```python
from build123d import *

# Parameters (mm, degrees)
EXTRUDE_1_DEPTH  = 11.2
SKETCH_3_W       = 40
SKETCH_3_H       = 20
EXTRUDE_2_DEPTH  = 5
EXTRUDE_3_DEPTH  = 10
EXTRUDE_4_DEPTH  = 5
SKETCH_7_W       = 98.8
SKETCH_7_H       = 34.24
EXTRUDE_5_DEPTH  = 9.8
SKETCH_8_W       = 80
SKETCH_8_H       = 34.24
EXTRUDE_6_DEPTH  = 5
SKETCH_9_W       = 35
SKETCH_9_H       = 30
EXTRUDE_7_DEPTH  = 5
EXTRUDE_8_DEPTH  = 40
FILLET_1_R       = 2
EXTRUDE_9_REACH  = 25.8
SKETCH_14_W      = 10
SKETCH_14_H      = 60
EXTRUDE_12_DEPTH = 167.8
EXTRUDE_13_DEPTH = 17.12
FILLET_3_R       = 2


with BuildPart() as part:
    # Sketch 1 → Extrude 1 (new body)
    with BuildSketch(Plane.XY):
        Polygon((0, 103.73), (5, 108.73), (95, 108.73), (100, 103.73), (100, 0), (0, 0), align=None)
    extrude(amount=EXTRUDE_1_DEPTH)



with BuildPart() as body_2:
    # Sketch 3 → Extrude 2 (new body)
    with BuildSketch(Plane.XY.offset(21.2)):
        with Locations((80, 86.29)):
            Rectangle(SKETCH_3_W, SKETCH_3_H)
    extrude(amount=EXTRUDE_2_DEPTH)


with BuildPart() as part_1:
    add(part.part)

    add(body_2.part)  # Extrude 3 merges body 2
    # Sketch 5 → Extrude 3 (add)
    with BuildSketch(Plane(origin=(0, 0, 21.2), x_dir=(-1, 0, 0), z_dir=(0, 0, -1))):
        Polygon((-60, 86.29), (-100, 81.29), (-100, 76.29), (-60, 76.29), align=None)
    extrude(amount=EXTRUDE_3_DEPTH)

    # Sketch 6 → Extrude 4 (add)
    with BuildSketch(Plane.ZY.offset(-60)):
        Polygon((26.2, 86.29), (155.2, 30), (155.2, 0), (26.2, 0), (11.2, 0), (11.2, 76.29), (26.2, 76.29), align=None)
    extrude(amount=-EXTRUDE_4_DEPTH)

    # Sketch 9 → Extrude 7 (add)
    with BuildSketch(Plane.XY.offset(155.2)):
        with Locations((82.5, 15)):
            Rectangle(SKETCH_9_W, SKETCH_9_H)
    extrude(amount=-EXTRUDE_7_DEPTH)



with BuildPart() as body_2_2:
    # Sketch 7 → Extrude 5 (new body)
    with BuildSketch(Plane.ZY.offset(-10.2)):
        with Locations((129.6, 17.12)):
            Rectangle(SKETCH_7_W, SKETCH_7_H)
    extrude(amount=-EXTRUDE_5_DEPTH)

    # Sketch 8 → Extrude 6 (add)
    with BuildSketch(Plane.XY.offset(179)):
        with Locations((60, 17.12)):
            Rectangle(SKETCH_8_W, SKETCH_8_H)
    extrude(amount=-EXTRUDE_6_DEPTH)


with BuildPart() as part_2:
    add(part_1.part)

    add(body_2_2.part)  # Extrude 8 merges body 2 2
    # Sketch 11 → Extrude 8 (add)
    with BuildSketch(Plane(origin=(20, 0, 0), x_dir=(0, 0, -1), z_dir=(1, 0, 0))):
        Polygon((-80.2, 0), (-80.2, 14), (-120.2, 17.12), (-174, 17.12), (-174, 0), align=None)
    extrude(amount=EXTRUDE_8_DEPTH)

    # Fillet 1
    fillet_1_edges = [part_2.edges().sort_by_distance(p)[0] for p in [
        (40, 14, 80.2),
    ]]
    fillet(fillet_1_edges, radius=FILLET_1_R)

    # Sketch 12 → Extrude 9 (add, up to next)
    with BuildSketch(Plane.XY.offset(155.2), mode=Mode.PRIVATE) as extrude_9_sk1:
        Polygon((60, 0), (60, 17.12), (100, 22), (100, 0), align=None)
    extrude_9_tool1 = extrude(extrude_9_sk1.sketch, amount=EXTRUDE_9_REACH, mode=Mode.PRIVATE) - part_2.part
    add(extrude_9_tool1.solids().sort_by_distance((80.831629, 9.830729, 155.2))[0])

    # Sketch 14 → Extrude 12 (add)
    with BuildSketch(Plane.XY.offset(11.2)):
        with Locations((5, 30)):
            Rectangle(SKETCH_14_W, SKETCH_14_H)
    extrude(amount=EXTRUDE_12_DEPTH)

    # Sketch 15 → Extrude 13 (add)
    with BuildSketch(Plane(origin=(0, 17.12, 0), x_dir=(1, 0, 0), z_dir=(0, 1, 0))):
        with BuildLine():
            Line((20, -159), (20, -174))
            Line((20, -174), (35, -174))
            ThreePointArc((35, -174), (24.393398282, -169.606601718), (20, -159))
        make_face()
    extrude(amount=EXTRUDE_13_DEPTH)

    # Fillet 3
    fillet_3_edges = [part_2.edges().sort_by_distance(p)[0] for p in [
        (60, 23.56, 155.2),
    ]]
    fillet(fillet_3_edges, radius=FILLET_3_R)


solid = part_2.part
```
For this review, take the finished solid that the model builds, in its own axes (mm). A direction names the side the tool comes from. Round coordinates to 2 decimals unless told otherwise and drop trailing zeros. Loops run counter-clockwise (first coordinate to the right, second up) from the corner with the lowest first, then second, coordinate; pieces in that order, holes last.
(1) We need section C-C (y = 55). Give the boundary of the cut face in (x, z).
Returned:
outline: (0, 0) - (100, 0) - (100, 11.2) - (65, 11.2) - (65, 97.91) - (60, 97.91) - (60, 11.2) - (10, 11.2) - (10, 179) - (0, 179) - close
(2) Clearance check with flat-ended pins moving along their axes: P1, Ø15, axis at x = 87, y = 15.5, coming from the -Z side; P2, Ø5, axis at x = 4.5, z = 124.5, coming from the +Y side; P3, Ø3, axis at y = 78, z = 41.5, coming from the -X side; P4, Ø6, axis at y = 31, z = 115.5, coming from the +X side. State where each tip first meets the part, or that it passes through.
Returned:
P1: stops at z = 0
P2: stops at y = 60
P3: stops at x = 60
P4: stops at x = 65
(3) Tool access review of faces 4 (the flat face through (82, 15, 150.2)), 5 (the flat face through (40, 67, 11.2)), 6 (the flat face through (29, 9, 80.2)), 7 (the flat face through (80, 91, 21.2)), 8 (the flat face through (5, 60, 94)): name each direction out of +Z, -Z, +X, -X, +Y, -Y from which nothing blocks a thin tool from reaching the whole face with its end or side.
Returned:
face 4: +X, +Y, -Y
face 5: +Y
face 6: +Y, -Y
face 7: +X, +Y
face 8: +Z, -X, +Y
(4) We need section D-D (z = 46). Give the boundary of the cut face in (x, y), plus the area to 3 significant figures.
Returned:
outline: (0, 0) - (10, 0) - (10, 60) - (0, 60) - close; (60, 0) - (65, 0) - (65, 77.65) - (60, 77.65) - close
area: 988 mm2
(5) Wall thickness on line 1 along Z through (x, y) = (75.5, 25); line 2 along X through (y, z) = (22.5, 145); line 3 along Z through (x, y) = (51, 11): over which ranges is each line inside the solid? List them lowest first.
Returned:
line 1: z = 0 to 11.2, 150.2 to 155.2, 174 to 179
line 2: x = 0 to 10, 10.2 to 20, 60 to 65
line 3: z = 0 to 11.2, 80.2 to 179
(6) Mouldability with a two-part tool opening along X and no side actions: class faces 1 (the flat face through (97.465, 106.265, 5.522)), 2 (the flat face through (39.72, 15.61, 100.86)), 3 (the flat face through (54, 17, 179)) as released by +X, released by -X, zero draft, split by the parting line, or undercut.
Returned:
face 1: released by +X
face 2: undercut
face 3: zero draft
(7) We need section B-B (z = 97). Give the boundary of the cut face in (x, y), plus the area to 3 significant figures.
Returned:
outline: (0, 0) - (10, 0) - (10, 60) - (0, 60) - close; (10.2, 0) - (65, 0) - (65, 55.4) - (60, 55.4) - (60, 15.31) - (20, 15.31) - (20, 34.24) - (10.2, 34.24) - close
area: 1,820 mm2
(8) We need section A-A (x = 47.5). Give the boundary of the cut face in (y, z), plus the area to 3 significant figures.
Returned:
outline: (0, 0) - (108.73, 0) - (108.73, 11.2) - (0, 11.2) - close; (0, 80.2) - (12.15, 80.2) arc R2 ccw to (14.14, 82.04) - (17.12, 120.2) - (17.12, 174) - (34.24, 174) - (34.24, 179) - (0, 179) - close
area: 2,930 mm2
